Here's how the part is built. I have some questions about the finished solid (model axes, mm). Give positions to 0.01 mm unless a question says otherwise; leave off trailing zeros. Loops run counter-clockwise (first coordinate to the right, second up) from the corner with the lowest first, then second, coordinate; pieces in that order, holes last. Notation, with made-up numbers: M -15.75,-21 L 25.25,-21 A17 ccw 25.25,0 Z; hole C 26,38 d8. An arc over 180 degrees is marked long. Answer as CSV lines item,"result". Start each with the question number.
Item 1: Will these pins go through, and if not, where does the flat tip stop? P1, Ø7.5, axis at x = -23.88, z = -32.09, coming from the -Y side; P2, Ø3, axis at y = 4.5, z = 206, coming from the -X side; P3, Ø1, axis at x = -32, y = 2, coming from the +Z side.
Item 2: I want a section at D-D on x = 41. List the corners of the cut face in (y, z) for me.
Item 3: I want a section at B-B on y = 2. List the corners of the cut face in (x, z) for me, plus the area to 3 significant figures.
Item 4: If I drill on line 1 along X through (y, z) = (0.75, 24.5); line 2 along X through (y, z) = (3, 44.5); line 3 along Z through (x, y) = (-23, 2.25), over which ranges is the centre line in solid material (lowest first)? Write a range as from..to.
Item 5: I want a section at C-C on z = 92. List the corners of the cut face in (x, y) for me, plus the area to 3 significant figures.
Item 6: I want a section at A-A on x = 0. List the corners of the cut face in (y, z) for me.
from build123d import *

# Parameters (mm, degrees)
EXTRUDE_1_DEPTH      = 6
SKETCH_6_R           = 3.25
CUT_EXTRUDE_3_DEPTH  = 28
CUT_EXTRUDE_11_DEPTH = 35


with BuildPart() as part:
    # 草图1 → 凸台-拉伸1 (new body)
    with BuildSketch(Plane(origin=(0, 0, 0), x_dir=(1, 0, 0), z_dir=(0, 1, 0))):
        with BuildLine():
            Line((-43.933694981, -23.871121576), (-72.986973894, -221.749637298))
            ThreePointArc((-72.986973894, -221.749637298), (-39.221926532, -267.135996225), (6.164432395, -233.370948863))
            Line((6.164432395, -233.370948863), (35.217711308, -35.492433141))
            ThreePointArc((35.217711308, -35.492433141), (7.263319728, 49.469628931), (-43.933694981, -23.871121576))
        make_face()
    extrude(amount=EXTRUDE_1_DEPTH)

    # 草图6 → 切除-拉伸3 (cut)
    with BuildSketch(Plane.XZ):
        with Locations(Location((-32.093002168, 23.87549396, 0), (0, 0, 270))):
            Circle(SKETCH_6_R)
        with Locations(Location((23.87549396, 32.093002168, 0), (0, 0, 270))):
            Circle(SKETCH_6_R)
        with Locations(Location((32.093002168, -23.87549396, 0), (0, 0, 270))):
            Circle(SKETCH_6_R)
        with Locations(Location((-23.87549396, -32.093002168, 0), (0, 0, 270))):
            Circle(SKETCH_6_R)
    extrude(amount=-CUT_EXTRUDE_3_DEPTH, mode=Mode.SUBTRACT)

    # 草图11 → 切除-拉伸11 (cut)
    with BuildSketch(Plane(origin=(0, 6, 0), x_dir=(1, 0, 0), z_dir=(0, 1, 0))):
        Polygon((9.713368511, 14.527342871), (11.529198442, 26.894750104), (11.10713535, 27.462079591), (-2.744360751, 29.495809113), (-3.311690238, 29.073746021), (-5.127520168, 16.706338788), (-3.4392678, 14.437020842), (7.444050565, 12.839090503), align=None)
    extrude(amount=-CUT_EXTRUDE_11_DEPTH, mode=Mode.SUBTRACT)


solid = part.part
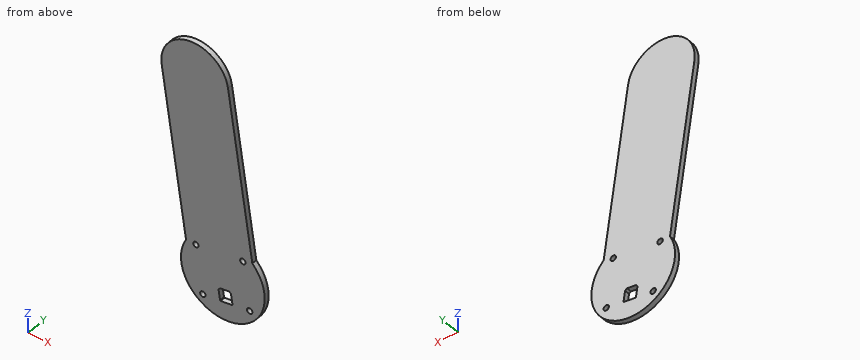
Result:
1,P1,"y = 0"
1,P2,"x = -70.89"
1,P3,"z = 267.55"
2,outline,"M 0,-28.62 L 6,-28.62 L 6,28.62 L 0,28.62 Z"
3,outline,"M -72.99,221.75 L -43.93,23.87 A50 ccw long 35.22,35.49 L 6.16,233.37 A40 ccw Z; hole C -32.09,23.88 d6.5; hole C -23.88,-32.09 d6.5; hole M -5.13,-16.71 L -3.31,-29.07 L -2.74,-29.5 L 11.11,-27.46 L 11.53,-26.89 L 9.71,-14.53 L 7.44,-12.84 L -3.44,-14.44 Z; hole C 23.88,32.09 d6.5; hole C 32.09,-23.88 d6.5"
3,area,"24,900 mm^2"
4,line 1,"-44.03..-35.28, -28.9..43.59"
4,line 2,"-46.96..33.9"
4,line 3,"-44.4..-35.22, -28.96..266.18"
5,outline,"M -53.94,0 L 26.92,0 L 26.92,6 L -53.94,6 Z"
5,area,"485 mm^2"
6,outline,"M 0,-50 L 6,-50 L 6,-29.09 L 0,-29.09 Z; M 0,-13.93 L 6,-13.93 L 6,249.55 L 0,249.55 Z"
